from build123d import *

# Parameters (mm, degrees)
SKETCH_1_W      = 19
SKETCH_1_H      = 8
SKETCH_1_R      = 1.7
EXTRUDE_1_DEPTH = 0.7
SKETCH_2_W      = 19
SKETCH_2_H      = 8
SKETCH_2_R      = 1.7
EXTRUDE_2_DEPTH = 0.7
FILLET_1_R      = 1
FILLET_2_R      = 0.25


with BuildPart() as part:
    # 草图1 → 凸台-拉伸1 (new body)
    with BuildSketch(Plane.XY):
        Rectangle(SKETCH_1_W, SKETCH_1_H)
        with Locations((-5.5, 0)):
            Circle(SKETCH_1_R, mode=Mode.SUBTRACT)
        with Locations((4.5, 0)):
            Circle(SKETCH_1_R, mode=Mode.SUBTRACT)
    extrude(amount=EXTRUDE_1_DEPTH)

    # 草图2 → 凸台-拉伸2 (add)
    with BuildSketch(Plane(origin=(9.5, 0, 0), x_dir=(0, 0, -1), z_dir=(1, 0, 0))):
        with Locations((-9.5, 0)):
            Rectangle(SKETCH_2_W, SKETCH_2_H)
        with Locations((-5, 0)):
            Circle(SKETCH_2_R, mode=Mode.SUBTRACT)
        with Locations((-15, 0)):
            Circle(SKETCH_2_R, mode=Mode.SUBTRACT)
    extrude(amount=-EXTRUDE_2_DEPTH)

    # 圆角1
    fillet_1_edges = [part.edges().sort_by_distance(p)[0] for p in [
        (9.15, 4, 19),
        (9.15, -4, 19),
        (-9.5, -4, 0.35),
        (-9.5, 4, 0.35),
    ]]
    fillet(fillet_1_edges, radius=FILLET_1_R)

    # 圆角2
    fillet_2_edges = [part.edges().sort_by_distance(p)[0] for p in [
        (9.5, 0, 0),
    ]]
    fillet(fillet_2_edges, radius=FILLET_2_R)


solid = part.part
Work out the finished part from the listing and answer in its coordinate system (mm). A direction names the side the tool comes from. Give positions to 0.01 mm unless a question says otherwise; leave off trailing zeros. Order: outer loops, then holes, each group sorted by start corner. A loop starts at its lowest first (then second) coordinate and runs counter-clockwise, first axis right, second up. Notation, with made-up numbers: (86.25, 61) -> (108.25, 61) arc R27 ccw to (108.25, 82) -> close; hole circle Ø7 at (-0.5, 19). An arc over 180 degrees is marked (long way). One line per item, written item: value.
Item 1: Flat-ended cylindrical pins translate along their axes: P1, Ø2.5, axis at x = 4.5, y = 0, coming from the -Z side; P2, Ø2.5, axis at x = 1.5, y = 1, coming from the +Z side. Find the tip coordinate at first contact, or state that the pin passes through.
Answer sheet:
P1: through
P2: z = 0.7
Item 2: Find section C-C, the plane z = 5. Give the vertices of the cut face in (x, y).
Answer sheet:
outline: (8.8, -4) -> (9.5, -4) -> (9.5, -1.7) -> (8.8, -1.7) -> close; (8.8, 1.7) -> (9.5, 1.7) -> (9.5, 4) -> (8.8, 4) -> close
Item 3: Straight lines are drawn through the part: probe 1 along Y at (x, z) = (4.5, 0.45); probe 2 along Z at (x, y) = (-2, 2.5); probe 3 along X at (y, z) = (0, 10). For each, find the intervals that lie inside material, in ascending order.
Answer sheet:
probe 1: -4 to -1.7, 1.7 to 4
probe 2: 0 to 0.7
probe 3: 8.8 to 9.5
Item 4: Find section D-D, the plane y = 2.75. Give the vertices of the cut face in (x, z), plus the area to 3 significant figures.
Answer sheet:
outline: (-9.5, 0) -> (9.25, 0) arc R0.25 ccw to (9.5, 0.25) -> (9.5, 19) -> (8.8, 19) -> (8.8, 0.7) -> (-9.5, 0.7) -> close
area: 26.1 mm²
Item 5: Determine the mould class of faces 3 (the cylindrical face through (-9.215, 3.699, 0.355)), 4 (the cylindrical face through (9.15, -0.65, 3.43)), 5 (the flat face through (8.8, 0, 10)) for opening direction Y: released by +Y, released by -Y, zero draft, split by the parting line, or undercut.
Answer sheet:
face 3: released by +Y
face 4: undercut
face 5: zero draft
Item 6: Find section B-B, the plane y = 0. Give the vertices of the cut face in (x, z).
Answer sheet:
outline: (-9.5, 0) -> (-7.2, 0) -> (-7.2, 0.7) -> (-9.5, 0.7) -> close; (-3.8, 0) -> (2.8, 0) -> (2.8, 0.7) -> (-3.8, 0.7) -> close; (6.2, 0) -> (9.25, 0) arc R0.25 ccw to (9.5, 0.25) -> (9.5, 3.3) -> (8.8, 3.3) -> (8.8, 0.7) -> (6.2, 0.7) -> close; (8.8, 6.7) -> (9.5, 6.7) -> (9.5, 13.3) -> (8.8, 13.3) -> close; (8.8, 16.7) -> (9.5, 16.7) -> (9.5, 19) -> (8.8, 19) -> close
Item 7: A tool of negligible diameter and unlimited length cuts with its end or side. For faces 1 (the flat face through (9.5, 0, 10)), 2 (the flat face through (0, 0, 0.7)), from which of +Z, -Z, +X, -X, +Y, -Y can it reach the whole face along a straight path? Write none if from no direction.
Answer sheet:
face 1: +Z, -Z, +X, +Y, -Y
face 2: +Z, -X, +Y, -Y
Item 8: Find section A-A, the plane x = 4.5. Give the vertices of the cut face in (y, z), plus the area to 3 significant figures.
Answer sheet:
outline: (-4, 0) -> (-1.7, 0) -> (-1.7, 0.7) -> (-4, 0.7) -> close; (1.7, 0) -> (4, 0) -> (4, 0.7) -> (1.7, 0.7) -> close
area: 3.22 mm²
